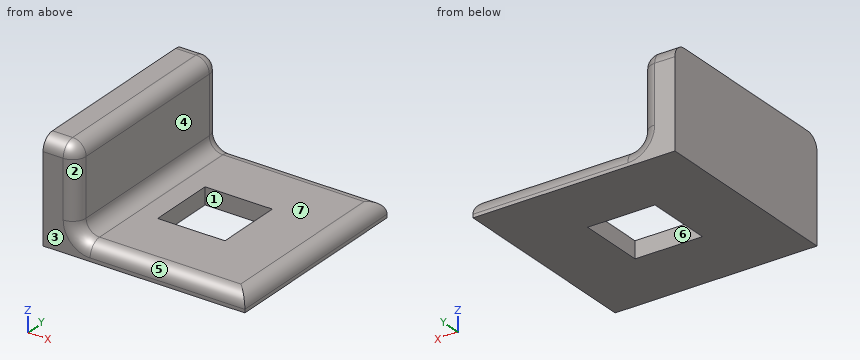
from build123d import *

# Parameters (mm, degrees)
F0_W     = 76.2
F0_H     = 76.2
F1_DEPTH = 6.35
F2_W     = 25.4
F2_H     = 25.4
F3_DEPTH = 25.4
F4_W     = 12.7
F4_H     = 76.2
F5_DEPTH = 31.75
F6_R     = 5.08
F7_R     = 5.08


with BuildPart() as f1:
    # F0 (on Top) → F1 (new body)
    with BuildSketch(Plane.XY):
        Rectangle(F0_W, F0_H)
    extrude(amount=F1_DEPTH)

    # F2 (on face) → F3 (cut)
    with BuildSketch(Plane.XY.offset(6.35)):
        Rectangle(F2_W, F2_H)
    extrude(amount=-F3_DEPTH, mode=Mode.SUBTRACT)

    # F4 (on face) → F5 (join)
    with BuildSketch(Plane.XY.offset(6.35)):
        with Locations((-31.75, 0)):
            Rectangle(F4_W, F4_H)
    extrude(amount=F5_DEPTH)

    # F6
    f6_edges = [f1.edges().sort_by_distance(p)[0] for p in [
        (-25.4, 0, 38.1),
        (-25.4, 0, 6.35),
    ]]
    fillet(f6_edges, radius=F6_R)

    # F7
    f7_edges = [f1.edges().sort_by_distance(p)[0] for p in [
        (8.89, -38.1, 6.35),
        (38.1, 0, 6.35),
        (8.89, 38.1, 6.35),
    ]]
    fillet(f7_edges, radius=F7_R)


solid = f1.part
Can you work these out from the model? Positions are in its coordinate system, mm. Face numbers are marked on the shaded views. A direction names the side the tool comes from. Round coordinates to 2 decimals unless told otherwise and drop trailing zeros. Write each loop counter-clockwise with the first axis right and the second up, starting at its lowest first coordinate (ties: lowest second). Pieces come first, ordered by that corner, then holes. Notation, with made-up numbers: (-35, -22) -> (22, -22) arc R35 ccw to (22, 10) -> close; hole circle Ø4 at (-17.5, -20). An arc over 180 degrees is marked (long way). Use one line per item in the form item = value. Start each with the question number.
Q1. I'm going to push flat-ended pins straight in: P1, Ø8, axis at x = -23.5, z = 25.5, coming from the -Y side; P2, Ø6, axis at x = -23, y = 25.5, coming from the -Z side; P3, Ø10, axis at y = 8.5, z = 30.5, coming from the +X side; P4, Ø1.9, axis at x = 4.5, z = 2.5, coming from the +Y side. Where does each tip first touch, or does it pass through?
Q2. Imagine slicing it at B-B (y = 2.5). Please give me the cut outline in (x, z).
Q3. Imagine slicing it at C-C (z = 14). Please give me the cut outline in (x, y), then the cut area to 3 significant figures.
Q4. If I drill on probe 1 along X at (y, z) = (-8, 32); probe 2 along Z at (x, y) = (4.5, -31); probe 3 along X at (y, z) = (-6, 35), over which ranges is the centre line in solid material (lowest first)? Write a range as [from, to].
Q5. Which directions (+Z, -Z, +X, -X, +Y, -Y) give clear straight access to the entire face, cutting with the end or side of a thin tool? Please do the marked faces 1, 2, 3 and 4.
Q6. We'd pull the mould along Y, two halves only. Please class the marked faces 5, 6 and 7: +Y half, -Y half, draft (parallel to the pull), parting line (faces both ways), or undercut.
Q7. Imagine slicing it at D-D (x = -18.5). Please give me the cut outline in (y, z), then the cut area to 3 significant figures.
Q8. Imagine slicing it at A-A (x = -4.5). Please give me the cut outline in (y, z), then the cut area to 3 significant figures.
Worked out:
q1.P1 = -37.13
q1.P2 = 0
q1.P3 = -25.4
q1.P4 = 38.09
q2.outline = (-38.1, 0) -> (-12.7, 0) -> (-12.7, 6.35) -> (-20.32, 6.35) arc R5.08 cw to (-25.4, 11.43) -> (-25.4, 33.02) arc R5.08 ccw to (-30.48, 38.1) -> (-38.1, 38.1) -> close; (12.7, 0) -> (38.1, 0) -> (38.1, 1.27) arc R5.08 ccw to (33.02, 6.35) -> (12.7, 6.35) -> close
q3.outline = (-38.1, -38.1) -> (-30.48, -38.1) arc R5.08 ccw to (-25.4, -33.02) -> (-25.4, 33.02) arc R5.08 ccw to (-30.48, 38.1) -> (-38.1, 38.1) -> close
q3.area = 957 mm^2
q4.probe_1 = [-38.1, -25.4]
q4.probe_2 = [0, 6.35]
q4.probe_3 = [-38.1, -25.8]
q5.face_1 = +Z, -Z
q5.face_2 = +Z, +X, -Y
q5.face_3 = +Z, -Z, +X, -X, -Y
q5.face_4 = +Z, +X, +Y, -Y
q6.face_5 = -Y half
q6.face_6 = undercut
q6.face_7 = draft
q7.outline = (-38.1, 0) -> (38.1, 0) -> (38.1, 1.27) arc R5.08 ccw to (33.02, 6.35) -> (-33.02, 6.35) arc R5.08 ccw to (-38.1, 1.27) -> close
q7.area = 473 mm^2
q8.outline = (-38.1, 0) -> (-12.7, 0) -> (-12.7, 6.35) -> (-33.02, 6.35) arc R5.08 ccw to (-38.1, 1.27) -> close; (12.7, 0) -> (38.1, 0) -> (38.1, 1.27) arc R5.08 ccw to (33.02, 6.35) -> (12.7, 6.35) -> close
q8.area = 312 mm^2
